from build123d import *

# Parameters (mm, degrees)
F1_DEPTH = 14
F3_DEPTH = 5
F4_R     = 2


with BuildPart() as f1:
    # F0 (on Front) → F1 (new body, symmetric)
    with BuildSketch(Plane.XZ):
        with BuildLine():
            ThreePointArc((-15, 0), (0, 15), (15, 0))
            Line((15, 0), (45, 0))
            Line((45, 0), (45, 25))
            Line((45, 25), (40, 25))
            Line((40, 25), (40, 5))
            Line((40, 5), (19.364916731, 5))
            ThreePointArc((19.364916731, 5), (-2.5200858497, 19.8405939253), (-20, 0))
            Line((-20, 0), (-15, 0))
        make_face()
    extrude(amount=F1_DEPTH, both=True)

    # F2 (on face) → F3 (cut, through all)
    with BuildSketch(Plane.YZ.offset(45)):
        with BuildLine():
            ThreePointArc((-4.5, 19.5), (-3.1819805217, 16.318019491), (-1.79e-08, 15))
            ThreePointArc((-1.79e-08, 15), (3.181980509, 16.3180194783), (4.5, 19.5))
            Line((4.5, 19.5), (4.5, 25))
            Line((4.5, 25), (-4.5, 25))
            Line((-4.5, 25), (-4.5, 19.5))
        make_face()
    extrude(amount=-F3_DEPTH, mode=Mode.SUBTRACT)

    # F4
    f4_edges = [f1.edges().sort_by_distance(p)[0] for p in [
        (42.5, -14, 25),
        (42.5, 14, 25),
    ]]
    fillet(f4_edges, radius=F4_R)


solid = f1.part
Source: CAD feature listing. Evaluate the final solid. Frame: model axes, mm. A direction names the side the tool comes from. Give positions to 0.01 mm unless a question says otherwise; leave off trailing zeros. Write each loop counter-clockwise with the first axis right and the second up, starting at its lowest first coordinate (ties: lowest second). Pieces come first, ordered by that corner, then holes. Notation, with made-up numbers: M 71.25,-17.5 L 82.25,-17.5 A35 ccw 82.25,18.5 Z; hole C 87.5,47.25 d11. An arc over 180 degrees is marked long. Answer as a JSON object with one key per item and string values.
Q1. Mould query, pull axis X, two halves, no side actions, for faces 1 (the face through (45, 0, 12)), 2 (the face through (42.46, -13.43, 24.4)), 3 (the face through (30, 0, 5)). Classes: +X half, -X half, draft (parallel to the pull), parting line (faces both ways), or undercut.
Geometry check:
{"face 1": "+X half", "face 2": "draft", "face 3": "undercut"}
Q2. Cut plane C-C, the plane x = 0. Return the cut outline in (y, z).
Geometry check:
{"outline": "M -14,15 L 14,15 L 14,20 L -14,20 Z"}
Q3. Cut plane A-A, the plane y = -7.25. Return the cut outline in (x, z).
Geometry check:
{"outline": "M -20,0 L -15,0 A15 cw 15,0 L 45,0 L 45,25 L 40,25 L 40,5 L 19.36,5 A20 ccw Z"}
Q4. Cut plane D-D, the plane z = 18. Return the cut outline in (x, y), then the cut area to 3 significant figures.
Geometry check:
{"outline": "M -8.72,-14 L 8.72,-14 L 8.72,14 L -8.72,14 Z; M 40,-14 L 45,-14 L 45,-4.24 L 40,-4.24 Z; M 40,4.24 L 45,4.24 L 45,14 L 40,14 Z", "area": "586 mm^2"}
Q5. Cut plane B-B, the plane z = 8.5. Return the cut outline in (x, y), then the cut area to 3 significant figures.
Geometry check:
{"outline": "M -18.1,-14 L -12.36,-14 L -12.36,14 L -18.1,14 Z; M 12.36,-14 L 18.1,-14 L 18.1,14 L 12.36,14 Z; M 40,-14 L 45,-14 L 45,14 L 40,14 Z", "area": "462 mm^2"}
Q6. Ray query, line 1 along X through (y, z) = (1, 8.5); line 2 along X through (y, z) = (-8.75, 12.5); line 3 along X through (y, z) = (13, 21.75). Return the intervals inside material, ascending.
Geometry check:
{"line 1": "x = -18.1 to -12.36, 12.36 to 18.1, 40 to 45", "line 2": "x = -15.61 to -8.29, 8.29 to 15.61, 40 to 45", "line 3": "x = 40 to 45"}
Q7. Access query for faces 4 (the face through (40, 0, 13)), 5 (the face through (42.46, 13.43, 24.4)). Directions: +Z, -Z, +X, -X, +Y, -Y. A direction counts if a zero-diameter tool reaches every point of the face in a straight line with its end or side. Return the directions, or none.
Geometry check:
{"face 4": "+Z, +Y, -Y", "face 5": "+Z, +X, -X, +Y"}
Q8. Contact query for flat-ended pins moving along their axis: P1, Ø2, axis at y = 4.5, z = 15.5, coming from the -X side (3 decimals); P2, Ø3, axis at y = -5, z = 13, coming from the -X side; P3, Ø4, axis at x = 22, y = 5.5, coming from the +Z side; P4, Ø5, axis at x = -9.5, z = 19, coming from the +Y side. Output: stop coordinate, or through.
Geometry check:
{"P1": "stops at x = -13.775", "P2": "stops at x = -16.36", "P3": "stops at z = 5", "P4": "stops at y = 14"}
